```python
from build123d import *

# Parameters (mm, degrees)
SKETCH_1_R               = 46
SKETCH_1_R_2             = 1.8
EXTRUDE_1_DEPTH          = 4
SKETCH_4_R               = 1.8
EXTRUDE_2_DEPTH          = 3
EXTRUDE_3_DEPTH          = 3
PATTERN_CIRCULAR_1_COUNT = 4
CUT_EXTRUDE_3_DEPTH      = 30
CUT_EXTRUDE_4_DEPTH      = 3
PATTERN_CIRCULAR_2_COUNT = 4
SKETCH_22_W              = 3
SKETCH_22_H              = 3
EXTRUDE_6_DEPTH          = 1
PATTERN_CIRCULAR_8_COUNT = 4
EXTRUDE_7_DEPTH          = 4
SKETCH_25_R              = 48
CUT_EXTRUDE_5_DEPTH      = 4


with BuildPart() as part:
    # Sketch 1 → Extrude 1 (new body)
    with BuildSketch(Plane.XY):
        with BuildLine():
            ThreePointArc((-17.648363843, -89.583265358), (0, -83.012821567), (17.648363843, -89.583265358))
            ThreePointArc((17.648363843, -89.583265358), (87.062445841, -87.062445841), (89.583265358, -17.648363843))
            ThreePointArc((89.583265358, -17.648363843), (83.012821567, 0), (89.583265358, 17.648363843))
            ThreePointArc((89.583265358, 17.648363843), (87.062445841, 87.062445841), (17.648363843, 89.583265358))
            ThreePointArc((17.648363843, 89.583265358), (0, 83.012821567), (-17.648363843, 89.583265358))
            ThreePointArc((-17.648363843, 89.583265358), (-87.062445841, 87.062445841), (-89.583265358, 17.648363843))
            ThreePointArc((-89.583265358, 17.648363843), (-83.012821567, 0), (-89.583265358, -17.648363843))
            ThreePointArc((-89.583265358, -17.648363843), (-87.062445841, -87.062445841), (-17.648363843, -89.583265358))
        make_face()
        with Locations((51, -51)):
            Circle(SKETCH_1_R, mode=Mode.SUBTRACT)
        with Locations((-51, -51)):
            Circle(SKETCH_1_R, mode=Mode.SUBTRACT)
        with BuildLine():
            ThreePointArc((-51, 0), (-65.702441614, -2.165194681), (-79.15650486, -8.476932918))
            ThreePointArc((-79.15650486, -8.476932918), (-78.012821567, 0), (-79.15650486, 8.476932918))
            ThreePointArc((-79.15650486, 8.476932918), (-65.702441614, 2.165194681), (-51, 0))
        make_face(mode=Mode.SUBTRACT)
        with Locations((-18.03122292, 0)):
            Circle(SKETCH_1_R_2, mode=Mode.SUBTRACT)
        with BuildLine():
            ThreePointArc((0, -51), (2.165194681, -65.702441614), (8.476932918, -79.15650486))
            ThreePointArc((8.476932918, -79.15650486), (0, -78.012821567), (-8.476932918, -79.15650486))
            ThreePointArc((-8.476932918, -79.15650486), (-2.165194681, -65.702441614), (0, -51))
        make_face(mode=Mode.SUBTRACT)
        with BuildLine():
            Line((-2.337899758, -28), (2.337899758, -28))
            ThreePointArc((2.337899758, -28), (4.008963141, -28.901115488), (4.174205427, -30.79245283))
            ThreePointArc((4.174205427, -30.79245283), (2.945040819, -33.920161063), (1.924528302, -37.122029053))
            ThreePointArc((1.924528302, -37.122029053), (0, -38.577794898), (-1.924528302, -37.122029053))
            ThreePointArc((-1.924528302, -37.122029053), (-2.945040819, -33.920161063), (-4.174205427, -30.79245283))
            ThreePointArc((-4.174205427, -30.79245283), (-4.008963141, -28.901115488), (-2.337899758, -28))
        make_face(mode=Mode.SUBTRACT)
        with Locations((0, -18.03122292)):
            Circle(SKETCH_1_R_2, mode=Mode.SUBTRACT)
        Polygon((9.899494937, 0), (0, -9.899494937), (-9.899494937, 0), (0, 9.899494937), align=None, mode=Mode.SUBTRACT)
        with Locations((18.03122292, 0)):
            Circle(SKETCH_1_R_2, mode=Mode.SUBTRACT)
        with BuildLine():
            Line((28, -2.337899758), (28, 2.337899758))
            ThreePointArc((28, 2.337899758), (28.901115488, 4.008963141), (30.79245283, 4.174205427))
            ThreePointArc((30.79245283, 4.174205427), (33.920161063, 2.945040819), (37.122029053, 1.924528302))
            ThreePointArc((37.122029053, 1.924528302), (38.577794898, 0), (37.122029053, -1.924528302))
            ThreePointArc((37.122029053, -1.924528302), (33.920161063, -2.945040819), (30.79245283, -4.174205427))
            ThreePointArc((30.79245283, -4.174205427), (28.901115488, -4.008963141), (28, -2.337899758))
        make_face(mode=Mode.SUBTRACT)
        with BuildLine():
            Line((-28, 2.337899758), (-28, -2.337899758))
            ThreePointArc((-28, -2.337899758), (-28.901115488, -4.008963141), (-30.79245283, -4.174205427))
            ThreePointArc((-30.79245283, -4.174205427), (-33.920161063, -2.945040819), (-37.122029053, -1.924528302))
            ThreePointArc((-37.122029053, -1.924528302), (-38.577794898, 0), (-37.122029053, 1.924528302))
            ThreePointArc((-37.122029053, 1.924528302), (-33.920161063, 2.945040819), (-30.79245283, 4.174205427))
            ThreePointArc((-30.79245283, 4.174205427), (-28.901115488, 4.008963141), (-28, 2.337899758))
        make_face(mode=Mode.SUBTRACT)
        with Locations((-51, 51)):
            Circle(SKETCH_1_R, mode=Mode.SUBTRACT)
        with Locations((0, 18.03122292)):
            Circle(SKETCH_1_R_2, mode=Mode.SUBTRACT)
        with BuildLine():
            ThreePointArc((1.924528302, 37.122029053), (2.945040819, 33.920161063), (4.174205427, 30.79245283))
            ThreePointArc((4.174205427, 30.79245283), (4.008963141, 28.901115488), (2.337899758, 28))
            Line((2.337899758, 28), (-2.337899758, 28))
            ThreePointArc((-2.337899758, 28), (-4.008963141, 28.901115488), (-4.174205427, 30.79245283))
            ThreePointArc((-4.174205427, 30.79245283), (-2.945040819, 33.920161063), (-1.924528302, 37.122029053))
            ThreePointArc((-1.924528302, 37.122029053), (0, 38.577794898), (1.924528302, 37.122029053))
        make_face(mode=Mode.SUBTRACT)
        with BuildLine():
            ThreePointArc((79.15650486, 8.476932918), (78.012821567, 0), (79.15650486, -8.476932918))
            ThreePointArc((79.15650486, -8.476932918), (65.702441614, -2.165194681), (51, 0))
            ThreePointArc((51, 0), (65.702441614, 2.165194681), (79.15650486, 8.476932918))
        make_face(mode=Mode.SUBTRACT)
        with BuildLine():
            ThreePointArc((-8.476932918, 79.15650486), (0, 78.012821567), (8.476932918, 79.15650486))
            ThreePointArc((8.476932918, 79.15650486), (2.165194681, 65.702441614), (0, 51))
            ThreePointArc((0, 51), (-2.165194681, 65.702441614), (-8.476932918, 79.15650486))
        make_face(mode=Mode.SUBTRACT)
        with Locations((51, 51)):
            Circle(SKETCH_1_R, mode=Mode.SUBTRACT)
    extrude(amount=EXTRUDE_1_DEPTH)

    # Sketch 8 → Extrude 3 (add, symmetric)
    with BuildSketch(Plane(origin=(0, 0, 0), x_dir=(0, 0, -1), z_dir=(1, 0, 0))):
        Polygon((23, 20.450291093), (23, 40.757425202), (4.692917013, 49.776091208), (0, 45.083174196), (0, 60.469008221), (4.692917013, 55.776091208), (26, 45.279527383), (26, 43.279527383), (26, 20.450291093), align=None)
    extrude_3 = extrude(amount=EXTRUDE_3_DEPTH, both=True)

    # Pattern Circular 1: Extrude 3 ×4 about axis
    pattern_circular_1_axis = Axis((0, 0, 0), (0, 0, 1))
    for i in range(1, PATTERN_CIRCULAR_1_COUNT):
        add(extrude_3.rotate(pattern_circular_1_axis, i * 360 / PATTERN_CIRCULAR_1_COUNT))

    # Sketch 12 → Cut-Extrude 3 (cut, symmetric)
    with BuildSketch(Plane.XY.offset(-23)):
        with BuildLine():
            Line((-19.798989873, -2.828427125), (-2.828427125, -19.798989873))
            ThreePointArc((-2.828427125, -19.798989873), (0, -20.970562748), (2.828427125, -19.798989873))
            Line((2.828427125, -19.798989873), (19.798989873, -2.828427125))
            ThreePointArc((19.798989873, -2.828427125), (20.970562748, 0), (19.798989873, 2.828427125))
            Line((19.798989873, 2.828427125), (2.828427125, 19.798989873))
            ThreePointArc((2.828427125, 19.798989873), (0, 20.970562748), (-2.828427125, 19.798989873))
            Line((-2.828427125, 19.798989873), (-19.798989873, 2.828427125))
            ThreePointArc((-19.798989873, 2.828427125), (-20.970562748, 0), (-19.798989873, -2.828427125))
        make_face()
    extrude(amount=CUT_EXTRUDE_3_DEPTH, both=True, mode=Mode.SUBTRACT)

    # Sketch 13 → Cut-Extrude 4 (cut)
    with BuildSketch(Plane(origin=(0, 0, -26), x_dir=(-1, 0, 0), z_dir=(0, 0, -1))):
        with BuildLine():
            Line((1.8, 33), (1.8, 31))
            ThreePointArc((1.8, 31), (0, 29.2), (-1.8, 31))
            Line((-1.8, 31), (-1.8, 33))
            ThreePointArc((-1.8, 33), (0, 34.8), (1.8, 33))
        make_face()
    cut_extrude_4 = extrude(amount=-CUT_EXTRUDE_4_DEPTH, mode=Mode.SUBTRACT)

    # Pattern Circular 2: Cut-Extrude 4 ×4 about axis
    pattern_circular_2_axis = Axis((0, 0, 0), (0, 0, 1))
    for i in range(1, PATTERN_CIRCULAR_2_COUNT):
        add(cut_extrude_4.rotate(pattern_circular_2_axis, i * 360 / PATTERN_CIRCULAR_2_COUNT), mode=Mode.SUBTRACT)



with BuildPart() as body_2:
    # Sketch 4 → Extrude 2 (new body)
    with BuildSketch(Plane.XY.offset(-26)):
        Polygon((-27.179581891, 0), (0, 27.179581891), (28.284271247, 0), (0, -28.284271247), align=None)
        with Locations((0, 18.03122292)):
            Circle(SKETCH_4_R, mode=Mode.SUBTRACT)
        with Locations((18.03122292, 0)):
            Circle(SKETCH_4_R, mode=Mode.SUBTRACT)
        with Locations((0, -18.03122292)):
            Circle(SKETCH_4_R, mode=Mode.SUBTRACT)
        with Locations((-18.03122292, 0)):
            Circle(SKETCH_4_R, mode=Mode.SUBTRACT)
    extrude(amount=EXTRUDE_2_DEPTH)


with BuildPart() as part_1:
    add(part.part)

    add(body_2.part)  # Extrude 6 merges body 2
    # Sketch 22 → Extrude 6 (add)
    with BuildSketch(Plane.ZY.offset(3)):
        with Locations((-24.5, 25.679581891)):
            Rectangle(SKETCH_22_W, SKETCH_22_H)
    extrude_6 = extrude(amount=-EXTRUDE_6_DEPTH)

    # Pattern Circular 8: Extrude 6 ×4 about axis
    pattern_circular_8_axis = Axis((0, 0, 0), (0, 0, -1))
    for i in range(1, PATTERN_CIRCULAR_8_COUNT):
        add(extrude_6.rotate(pattern_circular_8_axis, i * 360 / PATTERN_CIRCULAR_8_COUNT))

    # Sketch 24 → Extrude 7 (add)
    with BuildSketch(Plane.XY.offset(4)):
        with BuildLine():
            ThreePointArc((-68.748239349, 0), (-89.183766184, -89.183766184), (0, -68.748239349))
            ThreePointArc((0, -68.748239349), (89.183766184, -89.183766184), (68.748239349, 0))
            ThreePointArc((68.748239349, 0), (89.183766184, 89.183766184), (0, 68.748239349))
            ThreePointArc((0, 68.748239349), (-89.183766184, 89.183766184), (-68.748239349, 0))
        make_face()
        with BuildLine():
            Line((-5, 51), (5, 51))
            ThreePointArc((5, 51), (83.526911935, 83.526911935), (51, 5))
            Line((51, 5), (51, -5))
            ThreePointArc((51, -5), (83.526911935, -83.526911935), (5, -51))
            Line((5, -51), (-5, -51))
            ThreePointArc((-5, -51), (-83.526911935, -83.526911935), (-51, -5))
            Line((-51, -5), (-51, 5))
            ThreePointArc((-51, 5), (-83.526911935, 83.526911935), (-5, 51))
        make_face(mode=Mode.SUBTRACT)
    extrude(amount=-EXTRUDE_7_DEPTH)

    # Sketch 25 → Cut-Extrude 5 (cut)
    with BuildSketch(Plane.XY.offset(4)):
        with Locations((51, 51)):
            Circle(SKETCH_25_R)
        with Locations((51, -51)):
            Circle(SKETCH_25_R)
        with Locations((-51, -51)):
            Circle(SKETCH_25_R)
        with Locations((-51, 51)):
            Circle(SKETCH_25_R)
    extrude(amount=-CUT_EXTRUDE_5_DEPTH, mode=Mode.SUBTRACT)


solid = part_1.part
```
The listing builds one solid part. Answer for the finished solid, in the listing's coordinates (mm). A direction names the side the tool comes from. Give positions to 0.01 mm unless a question says otherwise; leave off trailing zeros. Order: outer loops, then holes, each group sorted by start corner. A loop starts at its lowest first (then second) coordinate and runs counter-clockwise, first axis right, second up. Notation, with made-up numbers: (-37.5, 31.25) -> (4.5, 31.25) arc R18 ccw to (4.5, 41.25) -> close; hole circle Ø8 at (21, -10.75). An arc over 180 degrees is marked (long way). Answer as CSV lines item,"result". Start each with the question number.
Q1. Which of the six approach directions +Z, -Z, +X, -X, +Y, -Y give full straight-line access (tool end or side, diameter ignored) to faces 1 (the flat face through (11.195, -11.433, 2.028)), 2 (the flat face through (47, 3, -14)), 3 (the flat face through (-0.042, -45.204, -13.975))?
Q2. Determine the mould class of faces 4 (the flat face through (-0.042, -47.462, -2.379)), 5 (the flat face through (-13.499, -14.236, -24.521)), 6 (the flat face through (0, 0, -23)), 7 (the flat face through (14.298, -13.986, -24.521)) for opening direction X: pulls with the +X half, pulls with the -X half, needs draft (parallel to the pull), parting line crosses it, or undercut.
Q3. Given pin 1 (8 mm diameter, centred on x = 19.5, z = -18.5, fed in from -Y); pin 2 (2 mm diameter, centred on y = -31.5, z = -24, fed in from +X); pin 3 (1.6 mm diameter, centred on y = 32.5, z = -24.5, fed in from -X); pin 4 (4 mm diameter, centred on x = -18.03, y = 0, fed in from +Z), each flat-ended and moving along its own axis, determine where each tip first touches the part or whether it passes through.
Q4. A cutting plane is placed at A-A (y = 63.5). Determine the outline of the cut face in (x, z).
Q5. Find the intervals of material crossed by L1, parallel to Y at x = 51, z = 1.4; L2, parallel to Y at x = 0, z = -25; L3, parallel to Z at x = 26, y = -9, in increasing order.
Q6. A cutting plane is placed at B-B (z = -14.5). Determine the outline of the cut face in (x, y).
Results found:
1,face 1,"+Z"
1,face 2,"-Z, +X, +Y"
1,face 3,"+X, -X"
2,face 4,"needs draft"
2,face 5,"pulls with the -X half"
2,face 6,"undercut"
2,face 7,"pulls with the +X half"
3,pin 1,"through"
3,pin 2,"x = 3"
3,pin 3,"x = -3"
3,pin 4,"z = -23"
4,outline,"(-103.53, 0) -> (-97.34, 0) -> (-97.34, 4) -> (-103.53, 4) -> close; (-4.66, 0) -> (4.66, 0) -> (4.66, 4) -> (-4.66, 4) -> close; (97.34, 0) -> (103.53, 0) -> (103.53, 4) -> (97.34, 4) -> close"
5,L1,"-105 to -99, -3 to 3, 99 to 105"
5,L2,"-45.77 to -34.8, -29.2 to -19.83, -16.23 to 16.23, 19.83 to 29.2, 34.8 to 45.77"
5,L3,"0 to 4"
6,outline,"(-50.94, -3) -> (-44.94, -3) -> (-44.94, 3) -> (-50.94, 3) -> close; (-3, -50.94) -> (3, -50.94) -> (3, -44.94) -> (-3, -44.94) -> close; (-3, 44.94) -> (3, 44.94) -> (3, 50.94) -> (-3, 50.94) -> close; (44.94, -3) -> (50.94, -3) -> (50.94, 3) -> (44.94, 3) -> close"
